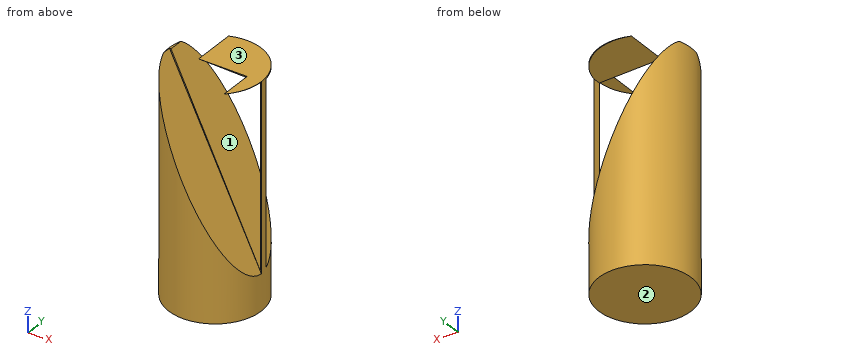
```python
from build123d import *

# Parameters (mm, degrees)
F0_R     = 25
F1_DEPTH = 120
F3_DEPTH = 25
F5_DEPTH = 145


with BuildPart() as f1:
    # F0 (on Top) → F1 (new body)
    with BuildSketch(Plane.XY):
        Circle(F0_R)
    extrude(amount=F1_DEPTH)

    # F2 (on Front) → F3 (cut)
    with BuildSketch(Plane.XZ):
        Polygon((25.316058, 119.865231), (-24.936564, 120.713368), (25.316058, 18.935909), align=None)
    extrude(amount=F3_DEPTH, mode=Mode.SUBTRACT)

    # F4 (on Front) → F5 (cut)
    with BuildSketch(Plane.XZ):
        Polygon((24.655644, 119.145423), (-23.93619, 120.385893), (24.655644, 20.490063), align=None)
    extrude(amount=-F5_DEPTH, mode=Mode.SUBTRACT)


solid = f1.part
```
Geometry check sheet. Reference: the model listing, model coordinates, mm. Face numbers are marked on the shaded views. Coordinates: 2 decimals unless noted, no trailing zeros. Write each loop counter-clockwise with the first axis right and the second up, starting at its lowest first coordinate (ties: lowest second). Pieces come first, ordered by that corner, then holes. Notation, with made-up numbers: M 49.5,22 L 72.5,22 A28 ccw 72.5,55 Z; hole C -0.5,10 d3. An arc over 180 degrees is marked long. One line per item, written item: value. Start each with the question number.
(1) Scan lines: line 1 along X through (y, z) = (0.5, 91) (3 decimals); line 2 along Z through (x, y) = (8.5, 20.5); line 3 along X through (y, z) = (2.5, 31). Record each from-to range of solid material in increasing order. Write a range as [from, to].
(2) Sectioned sample at D-D, the plane y = 2.5. Enter the section's corners in (x, z), and give its area (3 significant figures).
(3) Sectioned sample at C-C, the plane x = 13. Enter the section's corners in (y, z), and give its area (3 significant figures).
(4) Sectioned sample at B-B, the plane y = -11.5. Enter the section's corners in (x, z).
(5) Release check for a two-part mould opening along Z. For the marked faces 1, 2 and 3 record: released by +Z, released by -Z, zero draft, split by the parting line, or undercut.
(6) Depth check by flat-ended pin: pin 1 (3 mm diameter, centred on x = -11, y = 3, fed in from +Z); pin 2 (4.5 mm diameter, centred on y = 1, z = 91, fed in from -X); pin 3 (12 mm diameter, centred on y = -15.5, z = 46.5, fed in from -X); pin 4 (5 mm diameter, centred on y = -19, z = 27, fed in from +X). Enter the tip coordinate at first touch or a pass-through.
(7) Sectioned sample at A-A, the plane z = 73. Enter the section's corners in (x, y).
Filled sheet:
1. line 1: [-24.995, -9.642], [24.656, 24.995]
1. line 2: [0, 53.7], [119.56, 120]
1. line 3: [-24.87, 19.54], [24.66, 24.87]
2. outline: M -24.87,0 L 24.87,0 L 24.87,120 L -8.82,120 L 24.66,119.15 L 24.66,20.49 L -23.75,120 L -24.87,120 Z
2. area: 3,580 mm²
3. outline: M -21.35,0 L 21.35,0 L 21.35,44.45 L 0,44.45 L 0,43.88 L -21.35,43.88 Z; M 0,119.44 L 21.35,119.44 L 21.35,120 L 0,120 Z
3. area: 1,900 mm²
4. outline: M -22.2,0 L 22.2,0 L 22.2,25.25 L -22.2,115.17 Z; M 17.33,120 L 22.2,119.92 L 22.2,120 Z
5. face 1: undercut
5. face 2: released by -Z
5. face 3: released by +Z
6. pin 1: z = 96.88
6. pin 2: x = -25
6. pin 3: x = -23.12
6. pin 4: x = 18.78
7. outline: M -1.38,-24.96 L -1.38,0 L -0.89,0 L -0.89,24.98 A25 ccw Z; M 24.66,0 L 25,0 A25 ccw 24.66,4.14 Z
